Input: part model. Units: mm. Frame: model coordinates. Coordinates: 2 decimals unless noted, no trailing zeros. Order: outer loops, then holes, each group sorted by start corner. A loop starts at its lowest first (then second) coordinate and runs counter-clockwise, first axis right, second up. Notation, with made-up numbers: (89, -26.75) -> (125, -26.75) arc R34 ccw to (125, 10.25) -> close; hole circle Ø3 at (-26.75, 66.25). An arc over 180 degrees is marked (long way). One line per question, with ' | ' between items.
```python
from build123d import *

# Parameters (mm, degrees)
ESQUISSE1_W                  = 40
ESQUISSE1_H                  = 3
CHANFREIN1_SIZE              = 0.2
ESQUISSE2_R                  = 0.75
ENL_V_MAT_EXTRU_1_DEPTH      = 4
ENL_V_MAT_EXTRU_1_DEPTH_BACK = 4


with BuildPart() as part:
    # Esquisse1 → Révolution1 (revolve)
    with BuildSketch(Plane.XY):
        with Locations((5, 1.5)):
            Rectangle(ESQUISSE1_W, ESQUISSE1_H)
    revolve(axis=Axis((-15, 0, 0), (1, 0, 0)))

    # Chanfrein1
    chanfrein1_edges = [part.edges().sort_by_distance(p)[0] for p in [
        (-15, -3, 0),
        (25, -3, 0),
    ]]
    chamfer(chanfrein1_edges, length=CHANFREIN1_SIZE)

    # Esquisse2 → Enlèv. mat.-Extru.1 (cut, two sides)
    with BuildSketch(Plane.XY) as enl_v_mat_extru_1_sk:
        with Locations((-6.3, 0)):
            Circle(ESQUISSE2_R)
    extrude(amount=ENL_V_MAT_EXTRU_1_DEPTH, mode=Mode.SUBTRACT)
    extrude(enl_v_mat_extru_1_sk.sketch, amount=-ENL_V_MAT_EXTRU_1_DEPTH_BACK, mode=Mode.SUBTRACT)


solid = part.part
```
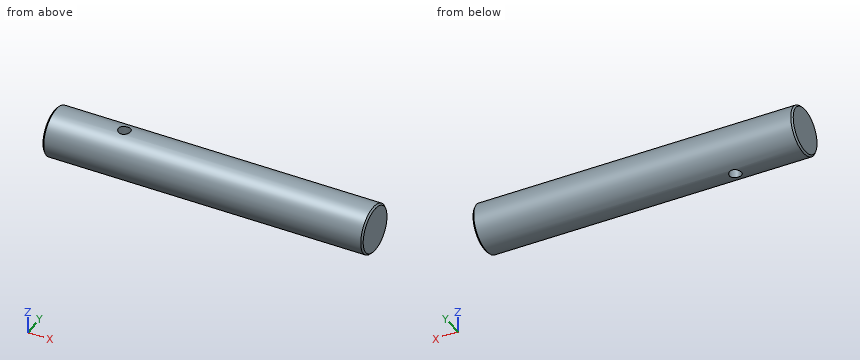
1. Cut plane A-A, the plane y = 0. Return loops of the section in (x, z).
Recorded:
outline: (-15, -2.8) -> (-14.8, -3) -> (-7.05, -3) -> (-7.05, 3) -> (-14.8, 3) -> (-15, 2.8) -> close; (-5.55, -3) -> (24.8, -3) -> (25, -2.8) -> (25, 2.8) -> (24.8, 3) -> (-5.55, 3) -> close
2. Cut plane B-B, the plane x = -6.3. Return loops of the section in (y, z).
Recorded:
outline: (-0.75, -2.9) -> (-0.75, 2.9) arc R3 ccw to start; (0.75, -2.9) arc R3 ccw to (0.75, 2.9) -> close
3. Cut plane C-C, the plane x = 11.5. Return loops of the section in (y, z).
Recorded:
outline: circle Ø6 at (0, 0)
4. Ray query, line 1 (X direction, y = 0, z = -1.4); line 2 (Y direction, x = -6.3, z = 2.35); line 3 (Y direction, x = -6.3, z = 1.95). Return the intervals inside material, ascending. Write a range as [from, to].
Recorded:
line 1: x = [-15, -7.05], [-5.55, 25] | line 2: y = [-1.86, -0.75], [0.75, 1.86] | line 3: y = [-2.28, -0.75], [0.75, 2.28]
5. Pin query (flat end, axial travel): pin 1 Ø1 at (x, y) = (5.5, 1.5) entering from +Z; pin 2 Ø1.5 at (x, y) = (-5.5, -1) entering from -Z; pin 3 Ø1.4 at (x, y) = (-6.3, 0) entering from +Z. Return the tip coordinate at first contact, or that it passes through.
Recorded:
pin 1: stops at z = 2.83 | pin 2: stops at z = -2.99 | pin 3: passes through
